from build123d import *

# Parameters (mm, degrees)
F1_DEPTH = 250
F4_R     = 5
F6_DEPTH = 25


with BuildPart() as f1:
    # F0 (on Top) → F1 (new body)
    with BuildSketch(Plane.XY):
        with BuildLine():
            Line((-75, 0), (0, 0))
            Line((0, 0), (0, 750))
            Line((0, 750), (-10, 750))
            ThreePointArc((-10, 750), (-58.7196001726, 376.4056986816), (-75, 0))
        make_face()
    extrude(amount=F1_DEPTH)

    # F2: F1 across face


with BuildPart() as f1_1:
    add(f1.part)
    add(f1.part.mirror(Plane(origin=(-37.5, 0, 125), x_dir=(1, 0, 0), z_dir=(0, -1, 0))))

    # F3: F1 across face


with BuildPart() as f1_2:
    add(f1_1.part)
    add(f1_1.part.mirror(Plane(origin=(0, 0, 125), x_dir=(0, 1, 0), z_dir=(1, 0, 0))))

    # F4
    f4_edges = [f1_2.edges().sort_by_distance(p)[0] for p in [
        (-10, -750, 125),
        (10, -750, 125),
        (10, 750, 125),
        (-10, 750, 125),
    ]]
    fillet(f4_edges, radius=F4_R)

    # F5 (on face) → F6 (join)
    with BuildSketch(Plane(origin=(0, 0, 0), x_dir=(1, 0, 0), z_dir=(0, 0, -1))):
        with BuildLine():
            ThreePointArc((35.3531478018, -750.1327120965), (100, 0), (35.3531478018, 750.1327120965))
            ThreePointArc((35.3531478018, 750.1327120965), (25.1089369329, 767.9562776043), (5.7954877704, 775))
            Line((5.7954877704, 775), (-5.7954877704, 775))
            ThreePointArc((-5.7954877704, 775), (-25.1089369329, 767.9562776043), (-35.3531478018, 750.1327120965))
            ThreePointArc((-35.3531478018, 750.1327120965), (-100, 0), (-35.3531478018, -750.1327120965))
            ThreePointArc((-35.3531478018, -750.1327120965), (-25.1089369329, -767.9562776043), (-5.7954877704, -775))
            Line((-5.7954877704, -775), (5.7954877704, -775))
            ThreePointArc((5.7954877704, -775), (25.1089369329, -767.9562776043), (35.3531478018, -750.1327120965))
        make_face()
    extrude(amount=-F6_DEPTH)


solid = f1_2.part
Can you work these out from the model? Positions are in its coordinate system, mm. A direction names the side the tool comes from. Give positions to 0.01 mm unless a question says otherwise; leave off trailing zeros. Order: outer loops, then holes, each group sorted by start corner. A loop starts at its lowest first (then second) coordinate and runs counter-clockwise, first axis right, second up. Notation, with made-up numbers: M 36.25,28.5 L 80.25,28.5 A25 cw 80.25,55.5 Z; hole C 61,-23 d2. An arc over 180 degrees is marked long. Use a Markdown table: item, result. Add a question column.
Item 1: Suppose I cut it at A-A (z = 144). List the corners of the cut face in (x, y) for me.
Item 2: Suppose I cut it at B-B (y = 209.5). List the corners of the cut face in (x, z) for me.
Item 3: If I drill on L1, parallel to Z at x = -82, y = -194; L2, parallel to X at y = -435, z = 224; L3, parallel to X at y = -274, z = 62, over which ranges is the centre line in solid material (lowest first)? Write a range as [from, to].
Item 4: For faces 1 (the cylindrical face through (-74.987, -10.494, 135.925)), 2 (the flat face through (81, -61, 25)), 3 (the cylindrical face through (74.987, -10.494, 135.925)), 4 (the cylindrical face through (24.883, 768.144, 12.325)), 5 (the cylindrical face through (25.33, -767.77, 12.32)), which set-ups out of +Z, -Z, +X, -X, +Y, -Y let a thin tool reach every point of the face, with its end or its side?
Item 5: Will these pins go through, and if not, where does the flat tip stop? pin 1 (9.5 mm diameter, centred on x = -0.5, z = 174.5, fed in from +Y); pin 2 (8 mm diameter, centred on x = -8.5, z = 111.5, fed in from -Y).
Answer sheet:
| question | item | result |
|---|---|---|
| 1 | outline | M -10.72,-745.86 A5 ccw -5.8,-750 L 5.8,-750 A5 ccw 10.72,-745.86 A4359.42 ccw 10.72,745.86 A5 ccw 5.8,750 L -5.8,750 A5 ccw -10.72,745.86 A4359.42 ccw Z |
| 2 | outline | M -94.99,0 L 94.99,0 L 94.99,25 L 69.96,25 L 69.96,250 L -69.96,250 L -69.96,25 L -94.99,25 Z |
| 3 | L1 | z = [0, 25] |
| 3 | L2 | x = [-53.24, 53.24] |
| 3 | L3 | x = [-66.38, 66.38] |
| 4 | face 1 | +Z, -X |
| 4 | face 2 | +Z |
| 4 | face 3 | +Z, +X |
| 4 | face 4 | +Z, -Z, +X, +Y |
| 4 | face 5 | +Z, -Z, +X, -Y |
| 5 | pin 1 | stops at y = 750 |
| 5 | pin 2 | stops at y = -750 |
